```python
from build123d import *

# Parameters (mm, degrees)
SKETCH1_W           = 278
SKETCH1_H           = 278
BOSS_EXTRUDE1_DEPTH = 6.35
SKETCH2_R           = 35
SKETCH2_R_2         = 2.75
CUT_EXTRUDE1_DEPTH  = 7.35
CHAMFER1_SIZE       = 20
SKETCH4_R           = 2.75
CUT_EXTRUDE2_DEPTH  = 76.2
SKETCH6_R           = 2.6
CUT_EXTRUDE4_DEPTH  = 7.35


with BuildPart() as part:
    # Sketch1 → Boss-Extrude1 (new body)
    with BuildSketch(Plane.XY):
        Rectangle(SKETCH1_W, SKETCH1_H)
    extrude(amount=BOSS_EXTRUDE1_DEPTH)

    # Sketch2 → Cut-Extrude1 (cut, through all)
    with BuildSketch(Plane.XY.offset(6.35)):
        Circle(SKETCH2_R)
        with Locations((-40, 40)):
            Circle(SKETCH2_R_2)
        with Locations((40, 40)):
            Circle(SKETCH2_R_2)
        with Locations((40, -40)):
            Circle(SKETCH2_R_2)
        with Locations((-40, -40)):
            Circle(SKETCH2_R_2)
    extrude(amount=-CUT_EXTRUDE1_DEPTH, mode=Mode.SUBTRACT)

    # Chamfer1
    chamfer1_edges = [part.edges().sort_by_distance(p)[0] for p in [
        (-139, 139, 3.175),
        (139, 139, 3.175),
        (139, -139, 3.175),
        (-139, -139, 3.175),
    ]]
    chamfer(chamfer1_edges, length=CHAMFER1_SIZE)

    # Sketch4 → Cut-Extrude2 (cut)
    with BuildSketch(Plane.XY.offset(6.35)):
        with Locations((-90, 130)):
            Circle(SKETCH4_R)
        with Locations((0, 130)):
            Circle(SKETCH4_R)
        with Locations((90, 130)):
            Circle(SKETCH4_R)
        with Locations((90, -130)):
            Circle(SKETCH4_R)
        with Locations((0, -130)):
            Circle(SKETCH4_R)
        with Locations((-90, -130)):
            Circle(SKETCH4_R)
    extrude(amount=-CUT_EXTRUDE2_DEPTH, mode=Mode.SUBTRACT)

    # Sketch6 → Cut-Extrude4 (cut, through all)
    with BuildSketch(Plane(origin=(0, 0, 0), x_dir=(-1, 0, 0), z_dir=(0, 0, -1))):
        with Locations((65, 65)):
            Circle(SKETCH6_R)
        with Locations((65, -65)):
            Circle(SKETCH6_R)
        with Locations((-65, -65)):
            Circle(SKETCH6_R)
        with Locations((-65, 65)):
            Circle(SKETCH6_R)
    extrude(amount=-CUT_EXTRUDE4_DEPTH, mode=Mode.SUBTRACT)


solid = part.part
```
Can you work these out from the model? Positions are in its coordinate system, mm. Give positions to 0.01 mm unless a question says otherwise; leave off trailing zeros. Loops run counter-clockwise (first coordinate to the right, second up) from the corner with the lowest first, then second, coordinate; pieces in that order, holes last. Notation, with made-up numbers: M 81,61.25 L 131,61.25 A10 ccw 131,67.25 Z; hole C -38.75,2.25 d4. An arc over 180 degrees is marked long. One line per question, with ' | ' between items. Start each with the question number.
Q1. If I drill on line 1 (Y direction, x = 90.5, z = 2.5); line 2 (X direction, y = -130, z = 4.75); line 3 (Y direction, x = -39, z = 1.5), over which ranges is the centre line in solid material (lowest first)? Write a range as from..to.
Q2. If we mould it in two halves opening along X, with no side actions, what happens to faces 1 (the flat face through (-2, 139, 3)), 2 (the cylindrical face through (-28, -21, 3)), 3 (the flat face through (-139, -2, 3))? For each: +X half, -X half, draft (parallel to the pull), parting line (faces both ways), or undercut.
Q3. If we section it at A-A (z = 3.75): State how many separate pieces and enclosed holes the cut face has, plus the area to 3 significant figures.
Q4. If we section it at B-B (y = -20.5): Please give me the cut outline in (x, z), plus the area to 3 significant figures.
Computed:
1) line 1: y = -139..-132.7, -127.3..127.3, 132.7..139 | line 2: x = -128..-92.75, -87.25..-2.75, 2.75..87.25, 92.75..128 | line 3: y = -139..-42.56, -37.44..37.44, 42.56..139
2) face 1: draft | face 2: undercut | face 3: -X half
3) separate pieces: 1 | enclosed holes: 15 | area: 72,300 mm²
4) outline: M -139,0 L -28.37,0 L -28.37,6.35 L -139,6.35 Z; M 28.37,0 L 139,0 L 139,6.35 L 28.37,6.35 Z | area: 1,410 mm²
